```python
from build123d import *

# Parameters (mm, degrees)
SKETCH1_R               = 3.175
EXTRUDE1_DEPTH          = 14.2875
EXTRUDE1_DEPTH_BACK     = 1.524
SKETCH2_R               = 4.826
EXTRUDE2_DEPTH          = 2.54
CHAMFER1_SIZE           = 0.508
CHAMFER2_SIZE           = 0.3175
SKETCH9_R               = 1.27
CUT_EXTRUDE1_DEPTH      = 3.175
CUT_EXTRUDE1_DEPTH_BACK = 3.175


with BuildPart() as part:
    # Sketch1 → Extrude1 (new body, two sides)
    with BuildSketch(Plane.XY) as extrude1_sk:
        Circle(SKETCH1_R)
    extrude(amount=EXTRUDE1_DEPTH)
    extrude(extrude1_sk.sketch, amount=-EXTRUDE1_DEPTH_BACK)

    # Sketch2 → Extrude2 (add)
    with BuildSketch(Plane.XY.offset(14.2875)):
        Circle(SKETCH2_R)
    extrude(amount=EXTRUDE2_DEPTH)

    # Chamfer1
    chamfer1_edges = [part.edges().sort_by_distance(p)[0] for p in [
        (-4.826, 0, 16.8275),
    ]]
    chamfer(chamfer1_edges, length=CHAMFER1_SIZE)

    # Chamfer2
    chamfer2_edges = [part.edges().sort_by_distance(p)[0] for p in [
        (-3.175, 0, -1.524),
    ]]
    chamfer(chamfer2_edges, length=CHAMFER2_SIZE)

    # Sketch9 → Cut-Extrude1 (cut, two sides)
    with BuildSketch(Plane(origin=(0, 0, 0), x_dir=(0, 0, -1), z_dir=(1, 0, 0))) as cut_extrude1_sk:
        with Locations((-7.9375, 0)):
            Circle(SKETCH9_R)
    extrude(amount=CUT_EXTRUDE1_DEPTH, mode=Mode.SUBTRACT)
    extrude(cut_extrude1_sk.sketch, amount=-CUT_EXTRUDE1_DEPTH_BACK, mode=Mode.SUBTRACT)


solid = part.part
```
Verification items for the finished model (mm, model axes). A direction names the side the tool comes from. Coordinates: 2 decimals unless noted, no trailing zeros. Order: outer loops, then holes, each group sorted by start corner. A loop starts at its lowest first (then second) coordinate and runs counter-clockwise, first axis right, second up. Notation, with made-up numbers: (61.25, 32) - (102.25, 32) arc R17 ccw to (102.25, 40) - close; hole circle Ø3 at (-39.75, 24.5). An arc over 180 degrees is marked (long way). Return JSON: item names as keys, results as strings.
(1) Go/stop test with flat-tipped pins: pin 1 (3 mm diameter, centred on y = 0, z = 7.94, fed in from +X) (3 decimals); pin 2 (5 mm diameter, centred on y = 3, z = 4.5, fed in from +X); pin 3 (5 mm diameter, centred on y = 2, z = 7.5, fed in from -X) (3 decimals). Record where each tip stops, or that it passes through.
Filled sheet:
{"pin 1": "stops at x = 3.175", "pin 2": "stops at x = 3.14", "pin 3": "stops at x = -3.175"}
(2) Section check B-B, the plane y = 0. Record the cut outline in (x, z) (1 decimal).
Filled sheet:
{"outline": "(-4.8, 14.3) - (-3.2, 14.3) - (-3.2, 9.2) - (3.2, 9.2) - (3.2, 14.3) - (4.8, 14.3) - (4.8, 16.3) - (4.3, 16.8) - (-4.3, 16.8) - (-4.8, 16.3) - close; (-3.2, -1.2) - (-2.9, -1.5) - (2.9, -1.5) - (3.2, -1.2) - (3.2, 6.7) - (-3.2, 6.7) - close"}
(3) Thickness scan on line 1 along Z through (x, y) = (-0.75, 0); line 2 along Z through (x, y) = (3, 1.25); line 3 along Z through (x, y) = (2, 1). Record the ranges inside material, lowest first.
Filled sheet:
{"line 1": "z = -1.52 to 6.67, 9.21 to 16.83", "line 2": "z = 14.29 to 16.83", "line 3": "z = -1.52 to 7.15, 8.72 to 16.83"}
(4) Section check D-D, the plane z = 4. Record the cut outline in (x, y) (3 decimals).
Filled sheet:
{"outline": "circle Ø6.35 at (0, 0)"}
(5) Mould release check, pull along Y, two halves, no side actions. Record for faces 3 (the cylindrical face through (0.044, 0.381, 6.726)), 4 (the cylindrical face through (-3.83, -2.937, 15.289)), 5 (the flat face through (0, 0, -1.524)): pulls with the +Y half, pulls with the -Y half, needs draft (parallel to the pull), parting line crosses it, or undercut.
Filled sheet:
{"face 3": "undercut", "face 4": "parting line crosses it", "face 5": "needs draft"}
(6) Section check C-C, the plane z = 14.5. Record the cut outline in (x, y).
Filled sheet:
{"outline": "circle Ø9.65 at (0, 0)"}
(7) Section check A-A, the plane x = 0. Record the cut outline in (y, z) (1 decimal).
Filled sheet:
{"outline": "(-4.8, 14.3) - (-3.2, 14.3) - (-3.2, -1.2) - (-2.9, -1.5) - (2.9, -1.5) - (3.2, -1.2) - (3.2, 14.3) - (4.8, 14.3) - (4.8, 16.3) - (4.3, 16.8) - (-4.3, 16.8) - (-4.8, 16.3) - close; hole circle Ø2.5 at (0, 7.9)"}
(8) Access from +Z, -Z, +X, -X, +Y, -Y to the whole of each face (thin tool, end or side, straight path). Record for faces 1 (the cylindrical face through (-0.69, -3.1, 6.65)), 2 (the flat face through (0, 0, 16.828)).
Filled sheet:
{"face 1": "-Z", "face 2": "+Z, +X, -X, +Y, -Y"}
